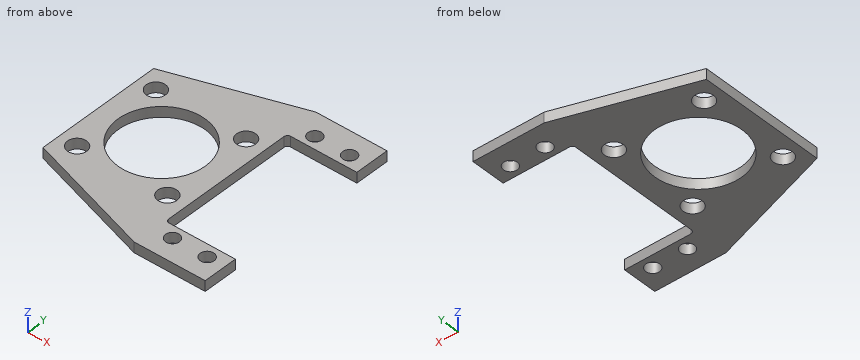
```python
from build123d import *

# Parameters (mm, degrees)
SKETCH1_R           = 2.75
SKETCH1_R_2         = 12.55
SKETCH1_R_3         = 2
BOSS_EXTRUDE1_DEPTH = 3


with BuildPart() as part:
    # Sketch1 → Boss-Extrude1 (new body)
    with BuildSketch(Plane(origin=(0, 0, 0), x_dir=(0, 1, 0), z_dir=(0, 0, 1))):
        with BuildLine():
            Line((-18.25, 18.25), (18.25, 18.25))
            Line((18.25, 18.25), (30, -18.25))
            Line((30, -18.25), (30, -38.75))
            Line((30, -38.75), (20.05, -38.75))
            Line((20.05, -38.75), (20.05, -19.65))
            ThreePointArc((20.05, -19.65), (19.757106781, -18.942893219), (19.05, -18.65))
            Line((19.05, -18.65), (-19.05, -18.65))
            ThreePointArc((-19.05, -18.65), (-19.757106781, -18.942893219), (-20.05, -19.65))
            Line((-20.05, -19.65), (-20.05, -38.75))
            Line((-20.05, -38.75), (-30, -38.75))
            Line((-30, -38.75), (-30, -18.25))
            Line((-30, -18.25), (-18.25, 18.25))
        make_face()
        with Locations(Location((-13, 13, 0), (0, 0, 270))):
            Circle(SKETCH1_R, mode=Mode.SUBTRACT)
        with Locations(Location((0, 0, 0), (0, 0, 270))):
            Circle(SKETCH1_R_2, mode=Mode.SUBTRACT)
        with Locations(Location((13, 13, 0), (0, 0, 270))):
            Circle(SKETCH1_R, mode=Mode.SUBTRACT)
        with Locations(Location((13, -13, 0), (0, 0, 270))):
            Circle(SKETCH1_R, mode=Mode.SUBTRACT)
        with Locations(Location((-13, -13, 0), (0, 0, 270))):
            Circle(SKETCH1_R, mode=Mode.SUBTRACT)
        with Locations(Location((-23.5, -23.65, 0), (0, 0, 270))):
            Circle(SKETCH1_R_3, mode=Mode.SUBTRACT)
        with Locations(Location((23.5, -23.65, 0), (0, 0, 270))):
            Circle(SKETCH1_R_3, mode=Mode.SUBTRACT)
        with Locations(Location((23.5, -33.65, 0), (0, 0, 270))):
            Circle(SKETCH1_R_3, mode=Mode.SUBTRACT)
        with Locations(Location((-23.5, -33.65, 0), (0, 0, 270))):
            Circle(SKETCH1_R_3, mode=Mode.SUBTRACT)
    extrude(amount=BOSS_EXTRUDE1_DEPTH)


solid = part.part
```
Geometry: final body of the model. Coordinates: model frame, mm. Give positions to 0.01 mm unless a question says otherwise; leave off trailing zeros. Loops run counter-clockwise (first coordinate to the right, second up) from the corner with the lowest first, then second, coordinate; pieces in that order, holes last. Notation, with made-up numbers: (-12, -23) -> (38, -23) arc R22 ccw to (38, 0) -> close; hole circle Ø6 at (61.25, 38). An arc over 180 degrees is marked (long way). Use one line per item in the form item = value.
Item 1: Pin query (flat end, axial travel): P1, Ø9, axis at x = 13, y = 13, coming from the +Z side; P2, Ø2, axis at x = 21.5, y = -8, coming from the +Z side; P3, Ø1.5, axis at y = -8, z = 2, coming from the +X side. Return the tip coordinate at first contact, or that it passes through.
A:
P1 = 3
P2 = through
P3 = 18.65
Item 2: Section query B-B on z = 0.65. Give the number of separate pieces and of enclosed holes in the cut face, and give its area (3 significant figures).
A:
separate_pieces = 1
enclosed_holes = 9
area = 1,550 mm^2
Item 3: Section query A-A on x = 23.65. Output: boundary loops of the cut face in (y, z).
A:
outline = (-30, 0) -> (-25.5, 0) -> (-25.5, 3) -> (-30, 3) -> close; (-21.5, 0) -> (-20.05, 0) -> (-20.05, 3) -> (-21.5, 3) -> close; (20.05, 0) -> (21.5, 0) -> (21.5, 3) -> (20.05, 3) -> close; (25.5, 0) -> (30, 0) -> (30, 3) -> (25.5, 3) -> close
Item 4: Section query D-D on x = 4. Output: boundary loops of the cut face in (y, z), and give its area (3 significant figures).
A:
outline = (-25.41, 0) -> (-11.9, 0) -> (-11.9, 3) -> (-25.41, 3) -> close; (11.9, 0) -> (25.41, 0) -> (25.41, 3) -> (11.9, 3) -> close
area = 81.1 mm^2
Item 5: Line query: probe 1 along Y at (x, z) = (23.65, 2.35); probe 2 along Y at (x, z) = (21.5, 1.3); probe 3 along Y at (x, z) = (13, 1.35). Output: solid intervals per line, ascending.
A:
probe_1 = -30 to -25.5, -21.5 to -20.05, 20.05 to 21.5, 25.5 to 30
probe_2 = -30 to -20.05, 20.05 to 30
probe_3 = -28.31 to -15.75, -10.25 to 10.25, 15.75 to 28.31
Item 6: Section query C-C on y = -4. Output: boundary loops of the cut face in (x, z).
A:
outline = (-18.25, 0) -> (-11.9, 0) -> (-11.9, 3) -> (-18.25, 3) -> close; (11.9, 0) -> (18.65, 0) -> (18.65, 3) -> (11.9, 3) -> close
